The model under review builds one solid part; all positions refer to its coordinate system, in mm. A direction names the side the tool comes from. Give positions to 0.01 mm unless a question says otherwise; leave off trailing zeros. Loops run counter-clockwise (first coordinate to the right, second up) from the corner with the lowest first, then second, coordinate; pieces in that order, holes last. Notation, with made-up numbers: M 45.25,68 L 76.25,68 A10 ccw 76.25,85 Z; hole C 37.5,46.5 d2. An arc over 180 degrees is marked long. Write item = value, one per line. Start each with the question number.
1. We need section C-C on x = 15. Give the boundary of the cut face in (y, z).
2. We need section A-A on z = 21. Give the boundary of the cut face in (x, y).
3. We need section B-B on y = 0. Give the boundary of the cut face in (x, z), then the cut area to 3 significant figures.
4. Draft analysis for pull direction Z (two halves, no side actions). For faces 4 (the face through (-25, 23, 14)), 5 (the face through (-25.5, 18.5, 12)), 6 (the face through (-23, -20, 15)), 7 (the face through (2, -20, 5)), state which applies: pulls with the +Z half, pulls with the -Z half, needs draft (parallel to the pull), parting line crosses it, or undercut.
5. For faces 1 (the face through (2, 15, 15)), 2 (the face through (13, 23, 3)), 3 (the face through (2, -15, 15)), list the 3-axis set-ups (+Z, -Z, +X, -X, +Y, -Y) from which the entire face can be reached by the end or side of a thin tool; tool diameter is ignored.
6. Wall thickness on line 1 along X through (y, z) = (6, 8); line 2 along Y through (x, z) = (-18, 22.5); line 3 along Z through (x, y) = (3.5, 22): over which ranges is each line inside the solid? List them lowest first. Write a range as from..to.
7. For pin 1 (6 mm diameter, centred on x = -10, z = 18, fed in from +Y); pin 2 (5 mm diameter, centred on y = 1.5, z = 21, fed in from +X); pin 3 (0.9 mm diameter, centred on y = 6, z = 23, fed in from -X); pin 4 (12 mm diameter, centred on x = 39.5, y = 17.5, fed in from -Z), all flat-tipped, find the tip position at first contact; note any pin that passes through.
8. We need section D-D on z = 15. Give the boundary of the cut face in (x, y), then the cut area to 3 significant figures.
from build123d import *

# Parameters (mm, degrees)
F0_W      = 56
F0_H      = 50
F1_DEPTH  = 5
F3_DEPTH  = 5
F4_W      = 5
F4_H      = 50
F5_DEPTH  = 17
F6_W      = 51
F6_H      = 30
F7_DEPTH  = 20
F9_DEPTH  = 5
F10_R     = 2
F11_DEPTH = 41


with BuildPart() as f1:
    # F0 (on Top) → F1 (new body)
    with BuildSketch(Plane.XY):
        Rectangle(F0_W, F0_H)
    extrude(amount=F1_DEPTH)

    # F2 (on face) → F3 (cut, through all)
    with BuildSketch(Plane.XY.offset(5)):
        with BuildLine():
            Line((17, -25), (17, -20.5))
            ThreePointArc((17, -20.5), (15, -18.5), (13, -20.5))
            Line((13, -20.5), (13, -25))
            Line((13, -25), (17, -25))
        make_face()
        with BuildLine():
            ThreePointArc((13, 20.5), (15, 18.5), (17, 20.5))
            Line((17, 20.5), (17, 25))
            Line((17, 25), (13, 25))
            Line((13, 25), (13, 20.5))
        make_face()
        with BuildLine():
            Line((-17, 25), (-17, 20.5))
            ThreePointArc((-17, 20.5), (-15, 18.5), (-13, 20.5))
            Line((-13, 20.5), (-13, 25))
            Line((-13, 25), (-17, 25))
        make_face()
        with BuildLine():
            ThreePointArc((-13, -20.5), (-15, -18.5), (-17, -20.5))
            Line((-17, -20.5), (-17, -25))
            Line((-17, -25), (-13, -25))
            Line((-13, -25), (-13, -20.5))
        make_face()
    extrude(amount=-F3_DEPTH, mode=Mode.SUBTRACT)

    # F4 (on face) → F5 (join)
    with BuildSketch(Plane.XY.offset(5)):
        with Locations((-25.5, 0)):
            Rectangle(F4_W, F4_H)
    extrude(amount=F5_DEPTH)

    # F6 (on face) → F7 (join)
    with BuildSketch(Plane.XY.offset(5)):
        with Locations((2.5, 0)):
            Rectangle(F6_W, F6_H)
    extrude(amount=F7_DEPTH)

    # F8 (on face) → F9 (cut, through all)
    with BuildSketch(Plane.YZ.offset(-23)):
        with BuildLine():
            Line((-25, 10), (-20.5, 10))
            ThreePointArc((-20.5, 10), (-18.5, 12), (-20.5, 14))
            Line((-20.5, 14), (-25, 14))
            Line((-25, 14), (-25, 10))
        make_face()
        with BuildLine():
            ThreePointArc((20.5, 14), (18.5, 12), (20.5, 10))
            Line((20.5, 10), (25, 10))
            Line((25, 10), (25, 14))
            Line((25, 14), (20.5, 14))
        make_face()
    extrude(amount=-F9_DEPTH, mode=Mode.SUBTRACT)

    # F10 (on face) → F11 (join)
    with BuildSketch(Plane.YZ.offset(28)):
        with Locations((0, 15)):
            Circle(F10_R)
    extrude(amount=F11_DEPTH)


solid = f1.part
Final values:
q1.outline = M -18.5,0 L 18.5,0 L 18.5,5 L 15,5 L 15,25 L -15,25 L -15,5 L -18.5,5 Z
q2.outline = M -28,-25 L -23,-25 L -23,-15 L 28,-15 L 28,15 L -23,15 L -23,25 L -28,25 Z
q3.outline = M -28,0 L 28,0 L 28,13 L 69,13 L 69,17 L 28,17 L 28,25 L -23,25 L -23,22 L -28,22 Z
q3.area = 1,550 mm²
q4.face_4 = undercut
q4.face_5 = undercut
q4.face_6 = needs draft
q4.face_7 = pulls with the +Z half
q5.face_1 = +Z, +X, +Y
q5.face_2 = +Z, -Z, +Y
q5.face_3 = +Z, +X, -Y
q6.line_1 = -28..28
q6.line_2 = -15..15
q6.line_3 = 0..5
q7.pin_1 = 15
q7.pin_2 = 28
q7.pin_3 = -23
q7.pin_4 = through
q8.outline = M -28,-25 L -23,-25 L -23,-15 L 28,-15 L 28,-2 L 69,-2 L 69,2 L 28,2 L 28,15 L -23,15 L -23,25 L -28,25 Z
q8.area = 1,940 mm²
